The model under review builds one solid part; all positions refer to its coordinate system, in mm. Face numbers are marked on the shaded views. A direction names the side the tool comes from. Round coordinates to 2 decimals unless told otherwise and drop trailing zeros. Write each loop counter-clockwise with the first axis right and the second up, starting at its lowest first coordinate (ties: lowest second). Pieces come first, ordered by that corner, then holes. Notation, with made-up numbers: (9.5, -9.75) -> (48.5, -9.75) arc R35 ccw to (48.5, 29.25) -> close; hole circle Ø4 at (63.5, -3). An arc over 180 degrees is marked (long way). Use CSV: the item, a comma, the result in double quotes. Start each with the question number.
1) Machinability: for the marked faces 1 and 2, which of the approach directions +Z, -Z, +X, -X, +Y, -Y give a long, thin tool a straight path to every point of the face, cutting with its end or side? Answer none if there is none.
2) Take a section at A-A, the plane y = 0. Give the boundary of the cut face in (x, z), then the cut area to 3 significant figures.
3) Wall thickness on probe 1 along Y at (x, z) = (-0.4, 21.5); probe 2 along Z at (x, y) = (0.3, -0.6); probe 3 along Z at (x, y) = (-1.7, -0.25): over which ranges is each line inside the solid? List them lowest first. Write a range as [from, to].
4) For pin 1 Ø1.5 at (x, z) = (1.5, 24.5) entering from +Y; pin 2 Ø0.8 at (x, y) = (0, 0.5) entering from -Z, all flat-tipped, find the tip position at first contact; note any pin that passes through.
5) Take a section at B-B, the plane z = 10. Give the boundary of the cut face in (x, y), then the cut area to 3 significant figures.
Autodesk Inventor part; units mm, degrees
ref_plane "YZ Plane" through (0, 0, 0) normal (1, 0, 0) x (0, 1, 0)
ref_plane "XZ Plane" through (0, 0, 0) normal (0, 1, 0) x (-1, 0, 0)
ref_plane "XY Plane" through (0, 0, 0) normal (0, 0, 1) x (1, 0, 0)
sketch "Sketch1" plane through (0, 0, 0) normal (0, 0, 1) x (1, 0, 0)
  circle A0 centre (0, 0) radius 1.5
  dimension "d0" = 3
extrude "Extrusion1" add sketch "Sketch1" along normal blind 28.8
thread "Thread1"
sketch "Sketch2" plane through (0, 0, 0) normal (0, 0, -1) x (-1, 0, 0)
  circle A0 centre (0, 0) radius 2
  dimension "d5" = 4
extrude "Extrusion2" add sketch "Sketch2" along normal blind 2
sketch "Sketch3" plane through (0, 0, -2) normal (0, 0, -1) x (-1, 0, 0)
  circle A0 centre (0, 0) radius 1.5
  line L0 (0, -1.4434) -> (-1.25, -0.7217)
  line L1 (-1.25, -0.7217) -> (-1.25, 0.7217)
  line L2 (-1.25, 0.7217) -> (0, 1.4434)
  line L3 (0, 1.4434) -> (1.25, 0.7217)
  line L4 (1.25, 0.7217) -> (1.25, -0.7217)
  line L5 (1.25, -0.7217) -> (0, -1.4434)
  dimension "d8" = 1.25
extrude "Extrusion3" cut sketch "Sketch3" against normal blind 1.5 contours L0 L1 L2 L3 L4 L5
fillet "Fillet1" radius 0.25 8 edges at (2, 0, 0) (2, 0, -2) (-0.625, -1.0825, -2) (-1.25, 0, -2) (-0.625, 1.0825, -2) (0.625, 1.0825, -2) (1.25, 0, -2) (0.625, -1.0825, -2)
properties part number "AdjBolt" material "Stainless Steel"
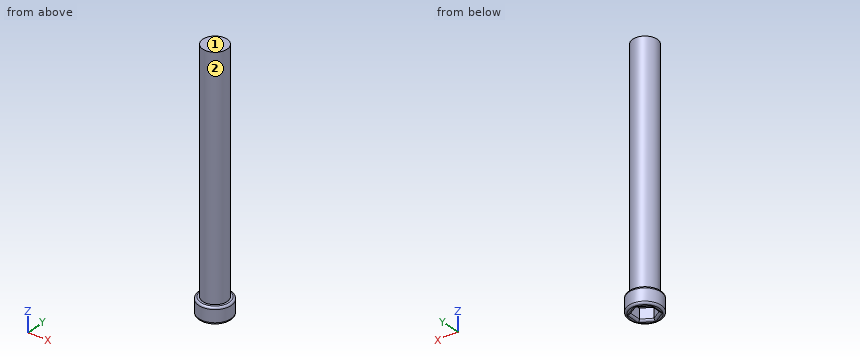
Values found:
1,face 1,"+Z, +X, -X, +Y, -Y"
1,face 2,"+Z"
2,outline,"(-2, -1.75) arc R0.25 ccw to (-1.75, -2) -> (-1.5, -2) arc R0.25 ccw to (-1.25, -1.75) -> (-1.25, -0.5) -> (1.25, -0.5) -> (1.25, -1.75) arc R0.25 ccw to (1.5, -2) -> (1.75, -2) arc R0.25 ccw to (2, -1.75) -> (2, -0.25) arc R0.25 ccw to (1.75, 0) -> (1.5, 0) -> (1.5, 28.8) -> (-1.5, 28.8) -> (-1.5, 0) -> (-1.75, 0) arc R0.25 ccw to (-2, -0.25) -> close"
2,area,"90.6 mm²"
3,probe 1,"[-1.45, 1.45]"
3,probe 2,"[-0.5, 28.8]"
3,probe 3,"[-2, 0]"
4,pin 1,"y = 1.3"
4,pin 2,"z = -0.5"
5,outline,"circle Ø3 at (0, 0)"
5,area,"7.07 mm²"
